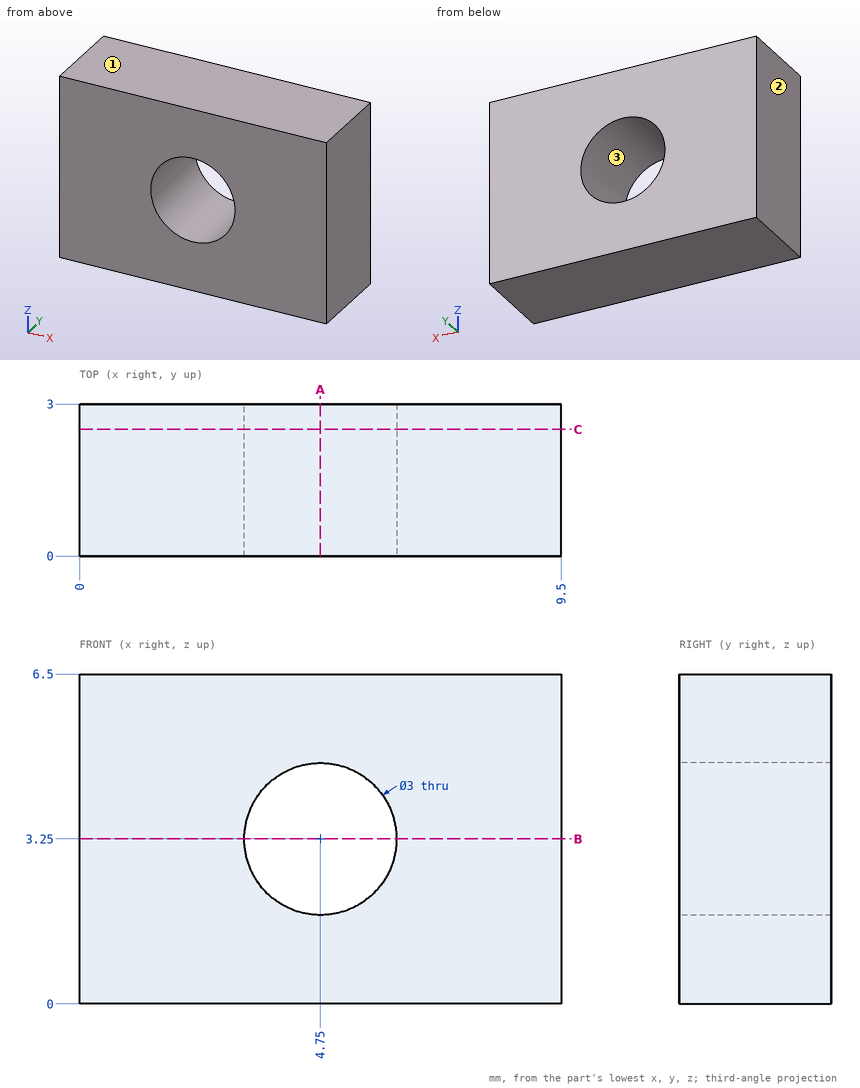
Could you check a few things on this drawing? It's one solid part, dimensions in mm from its lowest x, y, z. Round coordinates to 2 decimals unless told otherwise and drop trailing zeros. Loops run counter-clockwise (first coordinate to the right, second up) from the corner with the lowest first, then second, coordinate; pieces in that order, holes last. Notation, with made-up numbers: (35, 18) -> (89, 18) arc R21 ccw to (89, 28) -> close; hole circle Ø9 at (69.5, 76.25). An arc over 180 degrees is marked (long way). One line per item, written item: value. Start each with the question number.
1. If we section it at A-A, the plane x = 4.75: Write out the boundary of the cut face in (y, z).
2. If we section it at B-B, the plane z = 3.25: Write out the boundary of the cut face in (x, y).
3. If we section it at C-C, the plane y = 2.5: Write out the boundary of the cut face in (x, z).
4. If we mould it in two halves opening along Z, with no side actions, what happens to the marked faces 1, 2 and 3? For each: pulls with the +Z half, pulls with the -Z half, needs draft (parallel to the pull), parting line crosses it, or undercut.
5. If I drill on probe 1 along Z at (x, y) = (4.75, 1.95); probe 2 along X at (y, z) = (2.2, 3.5); probe 3 along X at (y, z) = (1.3, 4), over which ranges is the centre line in solid material (lowest first)?
Calculated:
1. outline: (0, 0) -> (3, 0) -> (3, 1.75) -> (0, 1.75) -> close; (0, 4.75) -> (3, 4.75) -> (3, 6.5) -> (0, 6.5) -> close
2. outline: (0, 0) -> (3.25, 0) -> (3.25, 3) -> (0, 3) -> close; (6.25, 0) -> (9.5, 0) -> (9.5, 3) -> (6.25, 3) -> close
3. outline: (0, 0) -> (9.5, 0) -> (9.5, 6.5) -> (0, 6.5) -> close; hole circle Ø3 at (4.75, 3.25)
4. face 1: pulls with the +Z half
4. face 2: needs draft
4. face 3: undercut
5. probe 1: z = 0 to 1.75, 4.75 to 6.5
5. probe 2: x = 0 to 3.27, 6.23 to 9.5
5. probe 3: x = 0 to 3.45, 6.05 to 9.5
